from build123d import *

# Parameters (mm, degrees)
BOSS_EXTRUDE1_DEPTH = 3
FILLET1_R           = 2


with BuildPart() as part:
    # Sketch2 → Boss-Extrude1 (new body)
    with BuildSketch(Plane.XY):
        with BuildLine():
            Line((4, 10.457560668), (4, -8.952439332))
            add(Edge.make_bspline(
                [(4, -8.952439332), (9.5, -9.387007233), (15, -10.717871431), (20.5, -12.945031924)],
                knots=[0.588888889, 0.588888889, 0.588888889, 0.588888889, 0.955555556, 0.955555556, 0.955555556, 0.955555556], degree=3))
            Line((20.5, -12.945031924), (20.5, 10.457560668))
            Line((20.5, 10.457560668), (4, 10.457560668))
        make_face()
    extrude(amount=-BOSS_EXTRUDE1_DEPTH)

    # Fillet1
    fillet1_edges = [part.edges().sort_by_distance(p)[0] for p in [
        (20.5, -12.945031924, -1.5),
        (4, -8.952439332, -1.5),
        (20.5, 10.457560668, -1.5),
        (4, 10.457560668, -1.5),
    ]]
    fillet(fillet1_edges, radius=FILLET1_R)


solid = part.part
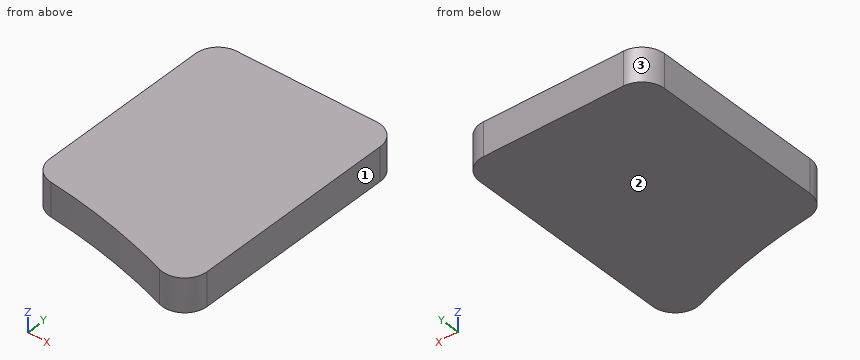
Geometry check sheet. Reference: the model listing, model coordinates, mm. Face numbers are marked on the shaded views. Round coordinates to 2 decimals unless told otherwise and drop trailing zeros.
Item 1: Material ranges on line 1 along X through (y, z) = (-8.25, -0.7); line 2 along Y through (x, z) = (15, -1.3); line 3 along Y through (x, z) = (9, -0.9), recorded low to high.
Determined:
line 1: x = 4.34 to 20.5
line 2: y = -11.02 to 10.46
line 3: y = -9.59 to 10.46
Item 2: Mould release check, pull along X, two halves, no side actions. Record for the marked faces 1, 2 and 3: +X half, -X half, draft (parallel to the pull), parting line (faces both ways), or undercut.
Determined:
face 1: +X half
face 2: draft
face 3: -X half
Item 3: Go/stop test with a flat-tipped pin: pin 1 Ø1.5 at (x, z) = (16.5, -2.5) entering from -Y. Record where the tip stops, or that it passes through.
Determined:
pin 1: stops at y = -11.73
